Model file for the job. Use its own axes, mm. A direction names the side the tool comes from. Round coordinates to 2 decimals unless told otherwise and drop trailing zeros. Order: outer loops, then holes, each group sorted by start corner. A loop starts at its lowest first (then second) coordinate and runs counter-clockwise, first axis right, second up. Notation, with made-up numbers: M 67.25,7.25 L 77.25,7.25 A21 cw 77.25,19.25 Z; hole C 87.5,-29 d5. An arc over 180 degrees is marked long. Return JSON: item names as keys, results as strings. Group by question number.
Item 1: Slice it at D-D on y = -17.5. Write the cut outline in (x, z) (1 decimal), then the cut area to 3 significant figures.
Item 2: Probe line 1 along Y through (x, z) = (12.7, 1.95); line 2 along Y through (x, z) = (0, 1.3); line 3 along X through (y, z) = (-9, 1.2) (3 decimals). List the from-to ranges inside material, lowest first.
Item 3: Slice it at B-B on z = 1.15. Give the number of separate pieces and of enclosed holes in the cut face, then the cut area to 3 significant figures.
Item 4: Slice it at A-A on x = 0. Write the cut outline in (y, z) (3 decimals).
Item 5: Pin check, flat tips, straight feed: pin 1 Ø1.6 at (x, z) = (-14.5, 1.5) entering from +Y; pin 2 Ø1.6 at (y, z) = (-8.5, 1) entering from +X (3 decimals); pin 3 Ø1 at (y, z) = (-8, 1.5) entering from -X (3 decimals); pin 4 Ø3.5 at (x, y) = (12.7, -28.194) entering from -Z. Stop position of each tip, or through.
Item 6: Pull direction Y, two halves, no side cores. Call faces 1 (the face through (-10.48, -14.59, 1.57)), 2 (the face through (-0.269, -30.246, 1.565)), 3 (the face through (20.638, -28, 2)): pulls with the +Y half, pulls with the -Y half, needs draft (parallel to the pull), parting line crosses it, or undercut.
Item 7: Slice it at C-C on y = -13. Write the cut outline in (x, z) (3 decimals).
Item 8: Which spindle directions (+Z, -Z, +X, -X, +Y, -Y) get a long thin tool onto all of the face, cutting with end or side? Do faces 4 (the face through (0, -24, 0)), 5 (the face through (9.525, -5, 2)). Say none if no direction does.
from build123d import *

# Parameters (mm, degrees)
SKETCH1_R           = 3.2004
SKETCH1_R_2         = 2.0701
BOSS_EXTRUDE1_DEPTH = 3.175
SKETCH2_W           = 33.106994052
SKETCH2_H           = 45.21414564
CUT_EXTRUDE1_DEPTH  = 46.916296315


with BuildPart() as part:
    # Sketch1 → Boss-Extrude1 (new body)
    with BuildSketch(Plane(origin=(0, 0, 0), x_dir=(-1, 0, 0), z_dir=(0, 0, -1))):
        with BuildLine():
            Line((-17.4625, -15.494), (-20.6375, -18.669))
            Line((-20.6375, -18.669), (-20.6375, -37.719))
            Line((-20.6375, -37.719), (-17.4625, -40.894))
            Line((-17.4625, -40.894), (17.4625, -40.894))
            Line((17.4625, -40.894), (20.6375, -37.719))
            Line((20.6375, -37.719), (20.6375, -18.669))
            Line((20.6375, -18.669), (17.4625, -15.494))
            Line((17.4625, -15.494), (12.7, -15.494))
            ThreePointArc((12.7, -15.494), (10.45493597, -14.56406403), (9.525, -12.319))
            Line((9.525, -12.319), (9.525, 1.2065))
            Line((9.525, 1.2065), (7.9375, 2.794))
            Line((7.9375, 2.794), (9.525, 4.3815))
            Line((9.525, 4.3815), (9.525, 37.719))
            Line((9.525, 37.719), (6.35, 40.894))
            Line((6.35, 40.894), (-6.35, 40.894))
            Line((-6.35, 40.894), (-9.525, 37.719))
            Line((-9.525, 37.719), (-9.525, 4.3815))
            Line((-9.525, 4.3815), (-7.9375, 2.794))
            Line((-7.9375, 2.794), (-9.525, 1.2065))
            Line((-9.525, 1.2065), (-9.525, -12.319))
            ThreePointArc((-9.525, -12.319), (-10.45493597, -14.56406403), (-12.7, -15.494))
            Line((-12.7, -15.494), (-17.4625, -15.494))
        make_face()
        with Locations(Location((0, 35.306, 0), (0, 0, 180))):
            Circle(SKETCH1_R, mode=Mode.SUBTRACT)
        with Locations(Location((0, -2.794, 0), (0, 0, 180))):
            Circle(SKETCH1_R, mode=Mode.SUBTRACT)
        with Locations(Location((12.7, -28.194, 0), (0, 0, 180))):
            Circle(SKETCH1_R_2, mode=Mode.SUBTRACT)
        with Locations(Location((-12.7, -28.194, 0), (0, 0, 180))):
            Circle(SKETCH1_R_2, mode=Mode.SUBTRACT)
        with Locations(Location((0, -28.194, 0), (0, 0, 180))):
            Circle(SKETCH1_R_2, mode=Mode.SUBTRACT)
    extrude(amount=-BOSS_EXTRUDE1_DEPTH)

    # Sketch2 → Cut-Extrude1 (cut, through all)
    with BuildSketch(Plane.XY.offset(3.175)):
        with Locations((5.708102423, 25.40107282)):
            Rectangle(SKETCH2_W, SKETCH2_H)
    extrude(amount=-CUT_EXTRUDE1_DEPTH, mode=Mode.SUBTRACT)


solid = part.part
Output values:
{
 "1": {"outline": "M -19.5,0 L 19.5,0 L 19.5,3.2 L -19.5,3.2 Z", "area": "124 mm²"},
 "2": {"line 1": "-40.89 to -30.26, -26.12 to -15.49", "line 2": "-40.89 to -30.26, -26.12 to -5.99, 0.41 to 2.79", "line 3": "-9.525 to 9.525"},
 "3": {"separate pieces": "1", "enclosed holes": "4", "area": "1,310 mm²"},
 "4": {"outline": "M -40.894,0 L -30.264,0 L -30.264,3.175 L -40.894,3.175 Z; M -26.124,0 L -5.994,0 L -5.994,3.175 L -26.124,3.175 Z; M 0.406,0 L 2.794,0 L 2.794,3.175 L 0.406,3.175 Z"},
 "5": {"pin 1": "y = -15.49", "pin 2": "x = 9.525", "pin 3": "x = -9.525", "pin 4": "through"},
 "6": {"face 1": "pulls with the +Y half", "face 2": "undercut", "face 3": "needs draft"},
 "7": {"outline": "M -9.599,0 L 9.599,0 L 9.599,3.175 L -9.599,3.175 Z"},
 "8": {"face 4": "-Z, +X, -X, +Y, -Y", "face 5": "+Z, -Z, +X, +Y"}
}
